CAD build for the part. Positions are in the model's coordinates, mm. A direction names the side the tool comes from. Give positions to 0.01 mm unless a question says otherwise; leave off trailing zeros. Loops run counter-clockwise (first coordinate to the right, second up) from the corner with the lowest first, then second, coordinate; pieces in that order, holes last. Notation, with made-up numbers: (-16.5, -27) -> (-7.5, -27) arc R24 ccw to (-7.5, 5) -> close; hole circle Ø2 at (52.25, -20). An arc over 180 degrees is marked (long way). Use one line per item in the form item = value.
```python
from build123d import *

# Parameters (mm, degrees)
F1_DEPTH = 1179
F2_W     = 260
F2_H     = 120
F3_DEPTH = 25
F5_DEPTH = 420
F7_DEPTH = 420
F9_DEPTH = 1200


with BuildPart() as f1:
    # F0 (on Right) → F1 (new body)
    with BuildSketch(Plane.YZ):
        Polygon((81, 4), (121, 0), (420, 0), (420, 3.2), (121.159602, 3.2), (81.159602, 7.2), (0, 7.2), (0, 4), align=None)
    extrude(amount=F1_DEPTH)

    # F2 (on face) → F3 (cut)
    with BuildSketch(Plane.XY.offset(3.2)):
        with Locations((455, 360)):
            Rectangle(F2_W, F2_H)
        with Locations((963, 360)):
            Rectangle(F2_W, F2_H)
    extrude(amount=-F3_DEPTH, mode=Mode.SUBTRACT)

    # F4 (on face) → F5 (join)
    with BuildSketch(Plane(origin=(0, 420, 0), x_dir=(-1, 0, 0), z_dir=(0, 1, 0))):
        Polygon((-17.771794, 1.599112), (-15, 0), (0, 26), (-2.771794, 27.599112), align=None)
    extrude(amount=-F5_DEPTH)

    # F6 (on face) → F7 (cut)
    with BuildSketch(Plane.XZ):
        Polygon((15, 0), (12.692308, 4), (0, 4), (0, 0), align=None)
        Polygon((12.692308, 4), (10.846154, 7.2), (0, 7.2), (0, 4), align=None)
    extrude(amount=-F7_DEPTH, mode=Mode.SUBTRACT)

    # F8 (on face) → F9 (cut)
    with BuildSketch(Plane.YZ.offset(1179)):
        Polygon((81, 4), (0, 4), (0, 0), (121, 0), align=None)
    extrude(amount=-F9_DEPTH, mode=Mode.SUBTRACT)


solid = f1.part
```
1. Drop flat-ended pins along their axis: P1, Ø8, axis at y = 86.5, z = 11.5, coming from the +X side; P2, Ø1.6, axis at y = 344, z = 1.5, coming from the -X side; P3, Ø4, axis at x = 760, y = 334, coming from the -Z side; P4, Ø12, axis at y = 212, z = 4.5, coming from the -X side. Give the stop position or say it passes through.
Result sheet:
P1 = 14.37
P2 = 13.67
P3 = 0
P4 = 8.94
2. Cut at A-A, the plane y = 346.5. Write the cut outline in (x, z).
Result sheet:
outline = (0, 26) -> (15, 0) -> (325, 0) -> (325, 3.2) -> (16.85, 3.2) -> (2.77, 27.6) -> close; (585, 0) -> (833, 0) -> (833, 3.2) -> (585, 3.2) -> close; (1093, 0) -> (1179, 0) -> (1179, 3.2) -> (1093, 3.2) -> close
3. Cut at B-B, the plane x = 388. Write the cut outline in (y, z).
Result sheet:
outline = (0, 4) -> (81, 4) -> (121, 0) -> (300, 0) -> (300, 3.2) -> (121.16, 3.2) -> (81.16, 7.2) -> (0, 7.2) -> close
4. Cut at C-C, the plane y = 149.5. Write the cut outline in (x, z).
Result sheet:
outline = (0, 26) -> (15, 0) -> (1179, 0) -> (1179, 3.2) -> (16.85, 3.2) -> (2.77, 27.6) -> close
5. Tool access for faces 1 (the flat face through (604, 41, 4)), 2 (the flat face through (589, 41, 7.2)), 3 (the flat face through (590, 239, 3.2)): list every direction of +Z, -Z, +X, -X, +Y, -Y with a clear straight run to the whole face (end or side of a thin tool).
Result sheet:
face_1 = -Z, +X, -X, -Y
face_2 = +Z, +X, +Y, -Y
face_3 = +Z, +X, +Y
6. Cut at D-D, the plane x = 613. Write the cut outline in (y, z), then the cut area to 3 significant figures.
Result sheet:
outline = (0, 4) -> (81, 4) -> (121, 0) -> (420, 0) -> (420, 3.2) -> (121.16, 3.2) -> (81.16, 7.2) -> (0, 7.2) -> close
area = 1,340 mm^2
7. Drill centre lines: line 1 (Z direction, x = 279, y = 80.5); line 2 (Z direction, x = 853.5, y = 175.5); line 3 (X direction, y = 103.5, z = 13.5). Where is each one in solid material? Low to high.
Result sheet:
line_1 = 4 to 7.2
line_2 = 0 to 3.2
line_3 = 7.21 to 10.91
